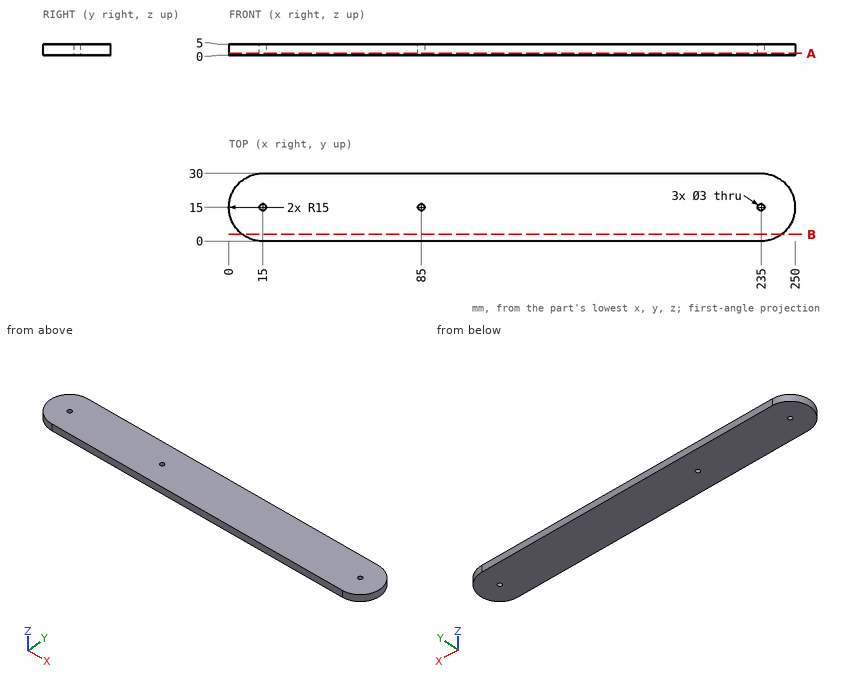
Answer from the drawing. Dimensions are ordinates in mm from the lowest x, y and z of the part. Round coordinates to 2 decimals unless told otherwise and drop trailing zeros. Write each loop counter-clockwise with the first axis right and the second up, starting at its lowest first coordinate (ties: lowest second). Pieces come first, ordered by that corner, then holes. Notation, with made-up numbers: M 31.25,26.25 L 89.25,26.25 A28 cw 89.25,65.25 Z; hole C 9.5,55 d6. An arc over 180 degrees is marked long. Write each question's results on one line, items separated by ' | '. Start each with the question number.
Item 1: Straight lines are drawn through the part: probe 1 along Y at (x, z) = (15, 1.9); probe 2 along X at (y, z) = (14, 0.55); probe 3 along X at (y, z) = (14.5, 0.4). For each, find the intervals that lie inside material, in ascending order.
Item 2: Given pin 1 Ø1.8 at (x, y) = (235, 15) entering from +Z; pin 2 Ø3 at (y, z) = (11.5, 4) entering from +X, each flat-ended and moving along its own axis, determine where each tip first touches the part or whether it passes through.
Item 3: Find section A-A on z = 0.85. Write down the section's boundary in (x, y).
Item 4: Find section B-B on y = 3. Write down the section's boundary in (x, z).
Answer block:
1) probe 1: y = 0 to 13.5, 16.5 to 30 | probe 2: x = 0.03 to 13.88, 16.12 to 83.88, 86.12 to 233.88, 236.12 to 249.97 | probe 3: x = 0.01 to 13.59, 16.41 to 83.59, 86.41 to 233.59, 236.41 to 249.99
2) pin 1: passes through | pin 2: stops at x = 249.87
3) outline: M 15,0 L 235,0 A15 ccw 235,30 L 15,30 A15 ccw Z; hole C 15,15 d3; hole C 85,15 d3; hole C 235,15 d3
4) outline: M 6,0 L 244,0 L 244,5 L 6,5 Z
